from build123d import *

# Parameters (mm, degrees)
CUT_EXTRUDE1_DEPTH      = 89.074065067
CUT_EXTRUDE1_DEPTH_BACK = 89.074065067
FILLET1_R               = 0.79375


with BuildPart() as part:
    # Sketch1 → Revolve1 (revolve)
    with BuildSketch(Plane.XY, mode=Mode.PRIVATE) as revolve1_sk:
        Polygon((-2.032, 0), (-2.032, 14.23435008), (-4.7625, 15.875), (-12.7, 15.875), (-12.7, 85.725), (-14.2875, 85.725), (-14.2875, 0), align=None)
    revolve(revolve1_sk.sketch.rotate(Axis((0, 0, 0), (0, 1, 0)), 270), axis=Axis((0, 0, 0), (0, 1, 0)))

    # Sketch2 → Cut-Extrude1 (cut, two sides: drawn at the far end of the back side and taken through both)
    with BuildSketch(Plane.XY.offset(-CUT_EXTRUDE1_DEPTH_BACK)):
        Polygon((-14.2875, 0), (14.2875, 13.324741332), (14.2875, 0), align=None)
    extrude(amount=CUT_EXTRUDE1_DEPTH + CUT_EXTRUDE1_DEPTH_BACK, mode=Mode.SUBTRACT)

    # Fillet1
    fillet1_edges = [part.edges().sort_by_distance(p)[0] for p in [
        (-10.102788136, 1.951363189, -10.102788136),
        (0, 85.725, 14.2875),
        (0, 85.725, 12.7),
        (0, 15.875, 12.7),
    ]]
    fillet(fillet1_edges, radius=FILLET1_R - 0.0001)  # a hair under: the kernel refuses the full size


solid = part.part
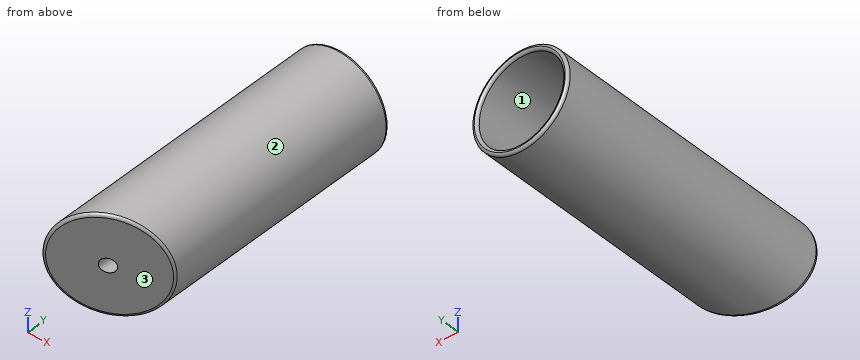
Geometry: final body of the model. Coordinates: model frame, mm. Face numbers are marked on the shaded views. Give positions to 0.01 mm unless a question says otherwise; leave off trailing zeros. Write each loop counter-clockwise with the first axis right and the second up, starting at its lowest first coordinate (ties: lowest second). Pieces come first, ordered by that corner, then holes. Notation, with made-up numbers: M 81,45 L 114,45 A17 cw 114,67 Z; hole C 43,85.25 d5. An arc over 180 degrees is marked long. Answer in a Markdown table with one row per item. Add a question column.
(1) Section A-A on y = 18.5. Return loops of the section in (x, z) (1 decimal), and give its area (3 significant figures).
(2) First-contact query: pin 1 (2 mm diameter, centred on y = 38.5, z = -8, fed in from +X); pin 2 (3 mm diameter, centred on y = 9.5, z = -5, fed in from -X); pin 3 (5 mm diameter, centred on y = 13.5, z = 10.5, fed in from +X). Flat tips, straight axial feed; report the tip coordinate or a pass-through.
(3) Mould query, pull axis X, two halves, no side actions, for the marked faces 1, 2 and 3. Classes: +X half, -X half, draft (parallel to the pull), parting line (faces both ways), or undercut.
(4) Ray query, line 1 (X direction, y = 43.5, z = 0); line 2 (Z direction, x = 11, y = 73); line 3 (Z direction, x = -3.5, y = 52). Return the intervals inside material, ascending.
Result set:
| question | item | result |
|---|---|---|
| 1 | outline | C 0,0 d28.6; hole C 0,0 d25.4 |
| 1 | area | 135 mm^2 |
| 2 | pin 1 | stops at x = 12.46 |
| 2 | pin 2 | stops at x = -13.85 |
| 2 | pin 3 | stops at x = 11.84 |
| 3 | face 1 | undercut |
| 3 | face 2 | parting line |
| 3 | face 3 | +X half |
| 4 | line 1 | x = -14.29 to -12.7, 12.7 to 14.29 |
| 4 | line 2 | z = -9.12 to -6.35, 6.35 to 9.12 |
| 4 | line 3 | z = -13.85 to -12.21, 12.21 to 13.85 |
